Check sheet for the modelled part. Datum: model origin and axes. Units: mm. A direction names the side the tool comes from. Give positions to 0.01 mm unless a question says otherwise; leave off trailing zeros. Order: outer loops, then holes, each group sorted by start corner. A loop starts at its lowest first (then second) coordinate and runs counter-clockwise, first axis right, second up.
```python
from build123d import *

# Parameters (mm, degrees)
F1_DEPTH    = 5
F2_W        = 10
F2_H        = 10
F3_DEPTH    = 13
F4_R        = 1
F5_W        = 5.5
F5_H        = 2
F7_DEPTH    = 11
F6_W        = 5.5
F6_H        = 2
F8_DEPTH    = 6
F9_T4_DEPTH = 30.5
F9_T7_DEPTH = 5.5


# Not quite as in the source:
# - a fillet or chamfer that OpenCascade refuses, or shapes differently, is made with other operations: its cross-section is extruded or revolved along the edge and cut away or added


with BuildPart() as f1:
    # F0 (on Top) → F1 (new body, symmetric)
    with BuildSketch(Plane.XY):
        Polygon((-6.777402997, 6.5974989831), (15.222597003, 6.5974989831), (15.222597003, 12.5974989831), (-12.777402997, 12.5974989831), (-12.777402997, -15.4025010169), (-6.777402997, -15.4025010169), align=None)
        Polygon((-8.777402997, -13.4025010169), (-10.777402997, -13.4025010169), (-10.777402997, 10.5974989831), (13.222597003, 10.5974989831), (13.222597003, 8.5974989831), (-8.777402997, 8.5974989831), align=None, mode=Mode.SUBTRACT)
    extrude(amount=F1_DEPTH, both=True)

    # F2 (on face) → F3 (join)
    with BuildSketch(Plane.XZ.offset(-6.5974989831)):
        with Locations((-1.777402997, 0)):
            Rectangle(F2_W, F2_H)
    extrude(amount=F3_DEPTH)

    # F4
    f4_edges = [f1.edges().sort_by_distance(p)[0] for p in [
        (3.222597, 6.597499, 0),
        (-12.777403, 12.597499, 0),
        (15.222597, 12.597499, 0),
        (15.222597, 6.597499, 0),
        (-12.777403, -15.402501, 0),
        (-6.777403, -15.402501, 0),
        (3.222597, -6.402501, 0),
        (-6.777403, -6.402501, 0),
    ]]
    fillet(f4_edges, radius=F4_R)

    # F5 (on face) → F7 (cut)
    with BuildSketch(Plane.XZ.offset(6.4025010169)):
        with Locations((-1.777402997, 0)):
            Rectangle(F5_W, F5_H)
    extrude(amount=-F7_DEPTH, mode=Mode.SUBTRACT)

    # F6 (on face) → F8 (cut, through all)
    with BuildSketch(Plane(origin=(0, 0, -5), x_dir=(1, 0, 0), z_dir=(0, 0, -1))):
        with Locations((-1.777402997, -3.5974989831)):
            Rectangle(F6_W, F6_H)
    extrude(amount=-F8_DEPTH, mode=Mode.SUBTRACT)

    # F9: fillet of radius 5 on 2 edges, made by hand


with BuildPart() as f9_tool2:
    # F9_s3 → F9_t4 (new body)
    with BuildSketch(Plane.YZ.offset(13.472597003)):
        with BuildLine():
            ThreePointArc((-0.4025010169, 1), (3.1330328891, -0.4644660941), (4.5974989831, -4))
            Line((4.5974989831, -4), (4.5974989831, 1))
            Line((4.5974989831, 1), (-0.4025010169, 1))
        make_face()
    extrude(amount=-F9_T4_DEPTH)

    split(bisect_by=Plane.YZ.offset(-8.777402997), keep=Keep.TOP)

    split(bisect_by=Plane.YZ.offset(3.222597003), keep=Keep.BOTTOM)


with BuildPart() as f1_1:
    add(f1.part)

    # F9_t1: union F9_tool2
    add(f9_tool2.part)

    # F9_s8 → F9_t7 (cut)
    with BuildSketch(Plane.YZ.offset(-4.527402997)):
        with BuildLine():
            ThreePointArc((2.5974989831, -5), (0.8607971577, -2.1270166538), (-2.3014805024, -1))
            Line((-2.3014805024, -1), (2.5974989831, -1))
            Line((2.5974989831, -1), (2.5974989831, -5))
        make_face()
    extrude(amount=F9_T7_DEPTH, mode=Mode.SUBTRACT)


solid = f1_1.part
```
(1) Set-up check for faces 1 (the face through (0.973, 0, -1)), 2 (the face through (14.937, 12.297, 0.07)), 3 (the face through (-1.8, 4.597, -4.5)), 4 (the face through (2, 8.597, 0)), 5 (the face through (-6.777, -11, 0)): record each of +Z, -Z, +X, -X, +Y, -Y from which the full face is reachable in a straight line by a thin tool's end or side.
Response values:
face 1: none
face 2: +Z, -Z, +X, +Y
face 3: -Z
face 4: +Z, -Z
face 5: +Z, -Z, +X, -Y
(2) Cross-section at A-A on y = 10. Enter the section's corners in (x, z), then the cut area to 3 significant figures.
Response values:
outline: (-12.78, -5) - (-10.78, -5) - (-10.78, 5) - (-12.78, 5) - close; (13.22, -5) - (15.22, -5) - (15.22, 5) - (13.22, 5) - close
area: 40.0 mm2
(3) Cross-section at C-C on x = -0.5. Enter the section's corners in (y, z), then the cut area to 3 significant figures.
Response values:
outline: (-6.4, -5) - (2.6, -5) arc R5 ccw to (-2.3, -1) - (-6.4, -1) - close; (-6.4, 1) - (-0.4, 1) arc R5 cw to (4.6, -4) - (4.6, -5) - (8.6, -5) - (8.6, 5) - (-6.4, 5) - close; (10.6, -5) - (12.6, -5) - (12.6, 5) - (10.6, 5) - close
area: 140 mm2
(4) Release check for a two-part mould opening along Z. For faces 6 (the face through (-1.82, 0.9, -2.16)), 7 (the face through (3.223, 0, 0)), 8 (the face through (-2, 2, -5)), 9 (the face through (-2, -3, 1)) record: released by +Z, released by -Z, zero draft, split by the parting line, or undercut.
Response values:
face 6: undercut
face 7: zero draft
face 8: released by -Z
face 9: undercut
(5) Cross-section at D-D on x = 9.25. Enter the section's corners in (y, z), then the cut area to 3 significant figures.
Response values:
outline: (6.6, -5) - (8.6, -5) - (8.6, 5) - (6.6, 5) - close; (10.6, -5) - (12.6, -5) - (12.6, 5) - (10.6, 5) - close
area: 40.0 mm2
(6) Gauge pin test, flat ends, axial feed: pin 1 Ø5 at (x, z) = (0, -0.5) entering from -Y; pin 2 Ø5.5 at (y, z) = (-11, -2) entering from +X; pin 3 Ø5 at (y, z) = (-0.5, -1.5) entering from +X. Record the tip position at first contact, or that the pin passes through.
Response values:
pin 1: stops at y = -6.4
pin 2: stops at x = -6.78
pin 3: stops at x = 3.22
(7) Cross-section at B-B on z = 1.75. Enter the section's corners in (x, y).
Response values:
outline: (-12.78, -14.4) arc R1 ccw to (-11.78, -15.4) - (-7.78, -15.4) arc R1 ccw to (-6.78, -14.4) - (-6.78, -7.4) arc R1 cw to (-5.78, -6.4) - (2.22, -6.4) arc R1 ccw to (3.22, -5.4) - (3.22, 5.6) arc R1 cw to (4.22, 6.6) - (14.22, 6.6) arc R1 ccw to (15.22, 7.6) - (15.22, 11.6) arc R1 ccw to (14.22, 12.6) - (-11.78, 12.6) arc R1 ccw to (-12.78, 11.6) - close; hole (-10.78, -13.4) - (-8.78, -13.4) - (-8.78, 8.6) - (13.22, 8.6) - (13.22, 10.6) - (-10.78, 10.6) - close
(8) Material ranges on L1, parallel to X at y = -4.75, z = -0.75; L2, parallel to X at y = -11.25, z = -2.75; L3, parallel to Y at x = 11.25, z = -3, recorded low to high.
Response values:
L1: x = -12.78 to -10.78, -8.78 to -4.53, 0.97 to 3.22
L2: x = -12.78 to -10.78, -8.78 to -6.78
L3: y = 6.6 to 8.6, 10.6 to 12.6
